Work out the finished part from the listing and answer in its coordinate system (mm). A direction names the side the tool comes from. Round coordinates to 2 decimals unless told otherwise and drop trailing zeros. Write each loop counter-clockwise with the first axis right and the second up, starting at its lowest first coordinate (ties: lowest second). Pieces come first, ordered by that corner, then holes. Notation, with made-up numbers: (47, 43.5) -> (83, 43.5) arc R22 ccw to (83, 70.5) -> close; hole circle Ø5 at (-4.75, 2.5). An arc over 180 degrees is marked (long way). One line per item, written item: value.
```python
from build123d import *

# Parameters (mm, degrees)
PAD040_DEPTH    = 90
SKETCH062_W     = 23.5
SKETCH062_H     = 19
POCKET016_DEPTH = 1.5
POCKET017_DEPTH = 5


with BuildPart() as part:
    # Sketch061 → Pad040 (new body, symmetric)
    with BuildSketch(Plane.XZ):
        Polygon((-1.5, 25), (-1.5, 1.5), (-25, 1.5), (-25, 0), (0, 0), (0, 25), align=None)
    extrude(amount=PAD040_DEPTH, both=True)

    # Sketch062 → Pocket016 (cut)
    with BuildSketch(Plane.XY):
        with Locations((-13.25, 80.5)):
            Rectangle(SKETCH062_W, SKETCH062_H)
    pocket016 = extrude(amount=POCKET016_DEPTH, mode=Mode.SUBTRACT)

    # Sketch063 → Pocket017 (cut)
    with BuildSketch(Plane.YZ):
        with BuildLine():
            ThreePointArc((75, 17.5), (70, 12.5), (75, 7.5))
            Line((75, 7.5), (90, 7.5))
            Line((90, 7.5), (90, 17.5))
            Line((90, 17.5), (75, 17.5))
        make_face()
    pocket017 = extrude(amount=-POCKET017_DEPTH, mode=Mode.SUBTRACT)

    # Mirrored018: Pocket017, Pocket016 across Sketch063 V_Axis
    add(pocket017.mirror(Plane(origin=(0, 0, 0), x_dir=(1, 0, 0), z_dir=(0, 1, 0))), mode=Mode.SUBTRACT)
    add(pocket016.mirror(Plane(origin=(0, 0, 0), x_dir=(1, 0, 0), z_dir=(0, 1, 0))), mode=Mode.SUBTRACT)


with BuildPart() as part_1:
    # Body031 placement: moved
    add(part.part.moved(Location((-136, 0, 0))))


solid = part_1.part
```
(1) Flat-ended cylindrical pins translate along their axes: pin 1 Ø12.5 at (y, z) = (-12, 8.5) entering from -X; pin 2 Ø1.5 at (x, y) = (-140, -38.5) entering from +Z; pin 3 Ø1.6 at (x, z) = (-145.5, 0.5) entering from +Y. Find the tip coordinate at first contact, or state that the pin passes through.
Reported:
pin 1: stops at x = -137.5
pin 2: stops at z = 1.5
pin 3: stops at y = 71
(2) For a pull along Z with two mould halves and no side action, classify faces 3 (the face through (-136, -1, 12)), 4 (the face through (-136.7, -70, 12.6)), 5 (the face through (-149, -1, 0)) as pulls with the +Z half, pulls with the -Z half, needs draft (parallel to the pull), parting line crosses it, or undercut.
Reported:
face 3: needs draft
face 4: undercut
face 5: pulls with the -Z half
(3) Find section B-B on z = 4.25. Give the vertices of the cut face in (x, y).
Reported:
outline: (-137.5, -90) -> (-136, -90) -> (-136, 90) -> (-137.5, 90) -> close
(4) A tool of negligible diameter and unlimited length cuts with its end or side. For faces 1 (the face through (-136.7, 70, 12.6)), 2 (the face through (-149, -1, 1.5)), from which of +Z, -Z, +X, -X, +Y, -Y can it reach the whole face along a straight path? Write none if from no direction.
Reported:
face 1: +X, -X, +Y
face 2: +Z, -X, +Y, -Y
(5) Find section C-C on x = -155. Give the vertices of the cut face in (y, z).
Reported:
outline: (-71, 0) -> (71, 0) -> (71, 1.5) -> (-71, 1.5) -> close
(6) Consider probe 1 along Z at (x, y) = (-149, -20); probe 2 along X at (y, z) = (50.5, 12). Determine where each line is inside the solid, lowest interval first.
Reported:
probe 1: z = 0 to 1.5
probe 2: x = -137.5 to -136
(7) Find section A-A on y = 25.5. Give the vertices of the cut face in (x, z), plus the area to 4 significant figures.
Reported:
outline: (-161, 0) -> (-136, 0) -> (-136, 25) -> (-137.5, 25) -> (-137.5, 1.5) -> (-161, 1.5) -> close
area: 72.75 mm2
